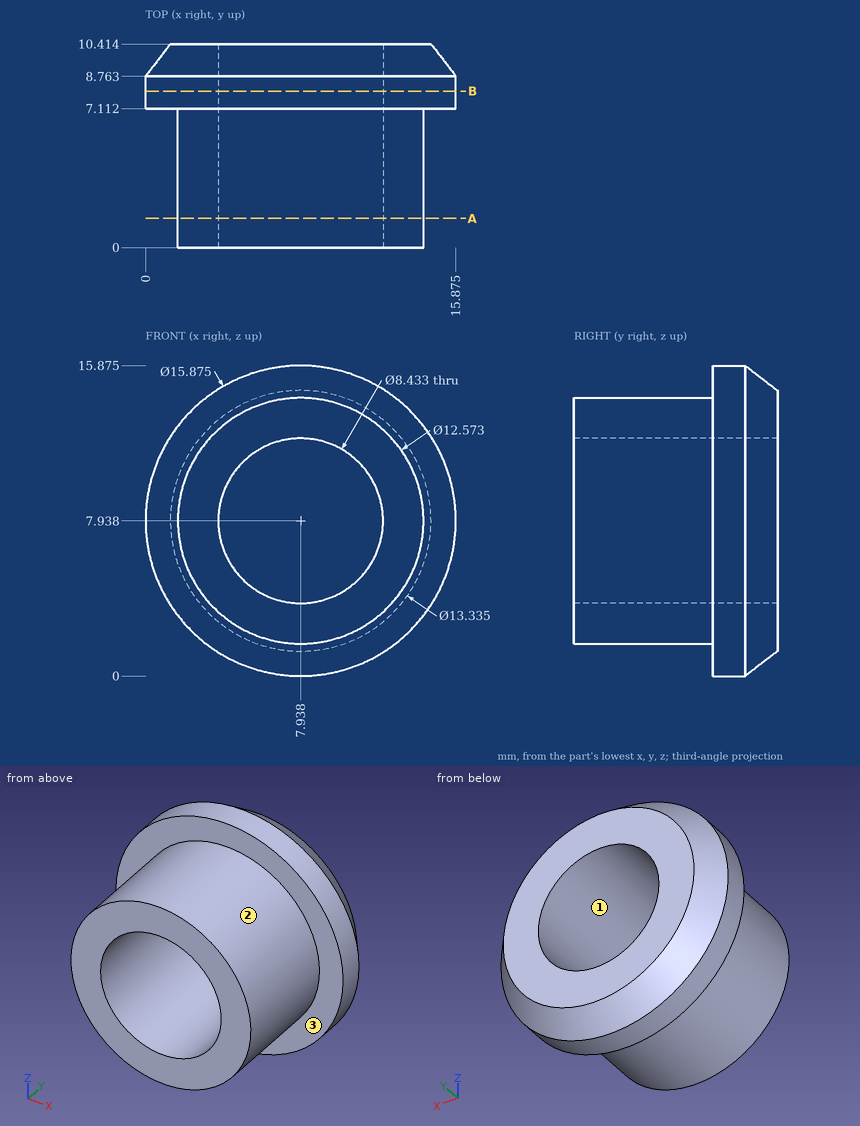
Study the drawing (mm; zero at the part's minimum x, y, z) and answer. Coordinates: 2 decimals unless noted, no trailing zeros. Write each loop counter-clockwise with the first axis right and the second up, starting at its lowest first coordinate (ties: lowest second). Pieces come first, ordered by that corner, then holes. Notation, with made-up numbers: (-30.5, -12.5) - (15.5, -12.5) arc R25 ccw to (15.5, 16.5) - close; hole circle Ø2 at (-13.5, 19). An arc over 180 degrees is marked (long way). Answer as a JSON object with one key per item and string values. Group by question number.
1. A cutting plane is placed at A-A (y = 1.5). Determine the outline of the cut face in (x, z) (1 decimal).
2. Each of these flat-tipped pins is pushed along its axis until it touches: P1, Ø6, axis at x = 6, y = 1, coming from the +Z side; P2, Ø3, axis at y = 3, z = 14, coming from the -X side; P3, Ø1.5, axis at x = 10.5, z = 7, coming from the +Y side; P4, Ø3, axis at y = 2.5, z = 12.5, coming from the -X side. Where does it stop, or does it pass through?
3. Consider L1, parallel to Z at x = 8.25, y = 3.5; L2, parallel to X at y = 7, z = 10 (1 decimal); L3, parallel to Z at x = 6.75, y = 5 (1 decimal). Determine where each line is inside the solid, lowest interval first. Write a range as [from, to].
4. The mould has two halves that part along X. Classify the marked faces 1, 2 and 3: +X half, -X half, draft (parallel to the pull), parting line (faces both ways), or undercut.
5. A cutting plane is placed at B-B (y = 8). Determine the outline of the cut face in (x, z) (1 decimal).
Worked out:
{
 "1": {"outline": "circle Ø12.6 at (7.9, 7.9); hole circle Ø8.4 at (7.9, 7.9)"},
 "2": {"P1": "stops at z = 14.22", "P2": "stops at x = 3.61", "P3": "passes through", "P4": "stops at x = 2.45"},
 "3": {"L1": "z = [1.66, 3.73], [12.14, 14.22]", "L2": "x = [2, 4.3], [11.6, 13.9]", "L3": "z = [1.8, 3.9], [12, 14.1]"},
 "4": {"face 1": "undercut", "face 2": "parting line", "face 3": "draft"},
 "5": {"outline": "circle Ø15.9 at (7.9, 7.9); hole circle Ø8.4 at (7.9, 7.9)"}
}
